from build123d import *

# Parameters (mm, degrees)
SKETCH_W        = 50
SKETCH_H        = 100
PAD_DEPTH       = 3
SKETCH001_R     = 1.6
POCKET_DEPTH    = 3
SKETCH002_R     = 1.6
POCKET001_DEPTH = 3
SKETCH003_R     = 3
POCKET002_DEPTH = 3
FILLET_R        = 1
FILLET001_R     = 2


with BuildPart() as part:
    # Sketch → Pad (new body)
    with BuildSketch(Plane.XY):
        Rectangle(SKETCH_W, SKETCH_H)
    extrude(amount=PAD_DEPTH)

    # Sketch001 (on Face6 of Pad) → Pocket (cut)
    with BuildSketch(Plane.XY.offset(3)):
        with Locations((-21, 46)):
            Circle(SKETCH001_R)
        with Locations((21, 46)):
            Circle(SKETCH001_R)
        with Locations((-21, -46)):
            Circle(SKETCH001_R)
        with Locations((21, -46)):
            Circle(SKETCH001_R)
    extrude(amount=-POCKET_DEPTH, mode=Mode.SUBTRACT)

    # Sketch002 (on Face5 of Pocket) → Pocket001 (cut)
    with BuildSketch(Plane.XY.offset(3)):
        with Locations((-12.5, 38)):
            Circle(SKETCH002_R)
        with Locations((12.5, 38)):
            Circle(SKETCH002_R)
        with Locations((-12.5, -26)):
            Circle(SKETCH002_R)
        with Locations((12.5, -26)):
            Circle(SKETCH002_R)
        Polygon((-15.5, 32), (-15.5, -20), (-7, -20), (-7, -28), (7, -28), (7, -20), (15.5, -20), (15.5, 32), (7, 32), (7, 40), (-7, 40), (-7, 32), align=None)
    extrude(amount=-POCKET001_DEPTH, mode=Mode.SUBTRACT)

    # Sketch003 (on Face5 of Pocket001) → Pocket002 (cut)
    with BuildSketch(Plane.XY.offset(3)):
        with Locations((16, -37)):
            Circle(SKETCH003_R)
    extrude(amount=-POCKET002_DEPTH, mode=Mode.SUBTRACT)

    # Fillet
    fillet_edges = [part.edges().sort_by_distance(p)[0] for p in [
        (25, -50, 1.5),
        (-25, -50, 1.5),
        (25, 50, 1.5),
        (-25, 50, 1.5),
    ]]
    fillet(fillet_edges, radius=FILLET_R)

    # Fillet001
    fillet001_edges = [part.edges().sort_by_distance(p)[0] for p in [
        (-7, 32, 1.5),
        (7, 32, 1.5),
        (-7, -20, 1.5),
        (7, -20, 1.5),
    ]]
    fillet(fillet001_edges, radius=FILLET001_R)


solid = part.part
Could you check a few things on this model? Use its own coordinates, in mm. A direction names the side the tool comes from. Give positions to 0.01 mm unless a question says otherwise; leave off trailing zeros. Loops run counter-clockwise (first coordinate to the right, second up) from the corner with the lowest first, then second, coordinate; pieces in that order, holes last. Notation, with made-up numbers: (-23.5, 1.25) -> (24.5, 1.25) arc R38 ccw to (24.5, 39.25) -> close; hole circle Ø9 at (-23.75, 16.5). An arc over 180 degrees is marked (long way). Answer as CSV lines item,"result". Start each with the question number.
(1) If we section it at B-B on z = 2.3: Count the separate pieces of the cut face and the enclosed holes in it, then the cut area to 3 significant figures.
(2) If we section it at A-A on y = -46: Write out the boundary of the cut face in (x, z), then the cut area to 3 significant figures.
(3) If we section it at C-C on x = 21: Write out the boundary of the cut face in (y, z).
(4) If we section it at D-D on y = -2: Write out the boundary of the cut face in (x, z).
(5) I need wall thicknesses on probe 1 along Y at (x, z) = (-21, 1.2); probe 2 along Y at (x, z) = (6, 0.9); probe 3 along Y at (x, z) = (-20, 1.8). Which ranges of each line are inside material? Lowest first, please.
(6) Which directions (+Z, -Z, +X, -X, +Y, -Y) give clear straight access to the entire face, cutting with the end or side of a thin tool? Please do faces 4 (the flat face through (-17, 1, 0)), 5 (the cylindrical face through (7.57, -20.6, 1.48)).
(7) We'd pull the mould along Y, two halves only. Please class faces 1 (the flat face through (0, 50, 1)), 2 (the flat face through (-25, -1, 1)), 3 (the cylindrical face through (-13.77, 37.03, 1.52)): released by +Y, released by -Y, zero draft, split by the parting line, or undercut.
Computed:
1,separate pieces,"1"
1,enclosed holes,"10"
1,area,"3,070 mm2"
2,outline,"(-25, 0) -> (-22.6, 0) -> (-22.6, 3) -> (-25, 3) -> close; (-19.4, 0) -> (19.4, 0) -> (19.4, 3) -> (-19.4, 3) -> close; (22.6, 0) -> (25, 0) -> (25, 3) -> (22.6, 3) -> close"
2,area,"131 mm2"
3,outline,"(-50, 0) -> (-47.6, 0) -> (-47.6, 3) -> (-50, 3) -> close; (-44.4, 0) -> (44.4, 0) -> (44.4, 3) -> (-44.4, 3) -> close; (47.6, 0) -> (50, 0) -> (50, 3) -> (47.6, 3) -> close"
4,outline,"(-25, 0) -> (-15.5, 0) -> (-15.5, 3) -> (-25, 3) -> close; (15.5, 0) -> (25, 0) -> (25, 3) -> (15.5, 3) -> close"
5,probe 1,"y = -50 to -47.6, -44.4 to 44.4, 47.6 to 50"
5,probe 2,"y = -50 to -28, 40 to 50"
5,probe 3,"y = -50 to -47.25, -44.75 to 44.75, 47.25 to 50"
6,face 4,"-Z, +X, -X, +Y, -Y"
6,face 5,"+Z, -Z"
7,face 1,"released by +Y"
7,face 2,"zero draft"
7,face 3,"undercut"
